Build history of the part. All positions in model axes, mm. A direction names the side the tool comes from. Round coordinates to 2 decimals unless told otherwise and drop trailing zeros. Write each loop counter-clockwise with the first axis right and the second up, starting at its lowest first coordinate (ties: lowest second). Pieces come first, ordered by that corner, then holes. Notation, with made-up numbers: (75.25, -32) - (101.25, -32) arc R15 cw to (101.25, -17) - close; hole circle Ø9 at (-35.75, 85.25). An arc over 180 degrees is marked (long way). One line per question, with ' | ' between items.
from build123d import *

# Parameters (mm, degrees)
SKETCH1_W               = 260
SKETCH1_H               = 150
SKETCH1_W_2             = 255
SKETCH1_H_2             = 145
BOSS_EXTRUDE1_DEPTH     = 110
SKETCH2_W               = 255
SKETCH2_H               = 145
BOSS_EXTRUDE2_DEPTH     = 2.5
SKETCH4_W               = 145
SKETCH4_H               = 2.5
BOSS_EXTRUDE3_DEPTH     = 45.5
CUT_EXTRUDE_THIN4_DEPTH = 5
SKETCH6_W               = 60
SKETCH6_H               = 30
CUT_EXTRUDE1_DEPTH      = 5
BOSS_EXTRUDE4_REACH     = 294.104
CUT_EXTRUDE2_DEPTH      = 3
SKETCH10_W              = 42.57
SKETCH10_H              = 23
CUT_EXTRUDE3_DEPTH      = 2.5
CUT_EXTRUDE4_DEPTH      = 2.5


with BuildPart() as part:
    # Sketch1 → Boss-Extrude1 (new body)
    with BuildSketch(Plane(origin=(0, 0, 0), x_dir=(1, 0, 0), z_dir=(0, 1, 0))):
        with Locations((130, 75)):
            Rectangle(SKETCH1_W, SKETCH1_H)
        with Locations((130, 75)):
            Rectangle(SKETCH1_W_2, SKETCH1_H_2, mode=Mode.SUBTRACT)
    extrude(amount=-BOSS_EXTRUDE1_DEPTH)

    # Sketch2 → Boss-Extrude2 (add)
    with BuildSketch(Plane(origin=(0, 0, 0), x_dir=(1, 0, 0), z_dir=(0, 1, 0))):
        with Locations((130, 75)):
            Rectangle(SKETCH2_W, SKETCH2_H)
    extrude(amount=-BOSS_EXTRUDE2_DEPTH)

    # Sketch4 → Boss-Extrude3 (add)
    with BuildSketch(Plane.ZY.offset(-257.5)):
        with Locations((-75, -93.15)):
            Rectangle(SKETCH4_W, SKETCH4_H)
    extrude(amount=BOSS_EXTRUDE3_DEPTH)

    # Sketch5 → Cut-Extrude-Thin4 (cut)
    with BuildSketch(Plane.XZ.offset(94.4)):
        Polygon((217.857864376, -60.857864376), (232, -75), (246.142135624, -60.857864376), (257.5, -60.857864376), (257.5, -60.858864376), (246.142549837, -60.858864376), (232, -75.001414214), (217.857157269, -60.858571483), align=None)
        with BuildLine():
            ThreePointArc((246.141113376, -60.858886624), (232, -55.001445677), (217.858886624, -60.858886624))
            Line((217.858886624, -60.858886624), (217.858179517, -60.858179517))
            ThreePointArc((217.858179517, -60.858179517), (232, -55.000445677), (246.141820483, -60.858179517))
            Line((246.141820483, -60.858179517), (246.141113376, -60.858886624))
        make_face()
    extrude(amount=-CUT_EXTRUDE_THIN4_DEPTH, mode=Mode.SUBTRACT)


with BuildPart() as cut_extrude_thin4_kept_piece:
    # of the separate pieces the step leaves, the one the design keeps (cut_extrude_thin4_pieces_kept)
    add(part.part.solids().sort_by_distance((0, 0, 0))[0])

    # Sketch6 → Cut-Extrude1 (cut)
    with BuildSketch(Plane(origin=(260, 0, 0), x_dir=(0, 0, -1), z_dir=(1, 0, 0))):
        with Locations((45, -78)):
            Rectangle(SKETCH6_W, SKETCH6_H)
    extrude(amount=-CUT_EXTRUDE1_DEPTH, mode=Mode.SUBTRACT)

    # Sketch8 → Boss-Extrude4 (add, up to next)
    with BuildSketch(Plane.XY.offset(-75), mode=Mode.PRIVATE) as boss_extrude4_sk1:
        Polygon((260, -63), (257.5, -64.647820306), (257.5, -63), align=None)
    boss_extrude4_tool1 = extrude(boss_extrude4_sk1.sketch, amount=BOSS_EXTRUDE4_REACH, mode=Mode.PRIVATE) - cut_extrude_thin4_kept_piece.part
    add(boss_extrude4_tool1.solids().sort_by_distance((258.333333, -63.549273, -75))[0])

    # Sketch9 → Cut-Extrude2 (cut)
    with BuildSketch(Plane.XZ.offset(94.4)):
        with BuildLine():
            Line((232, -75), (246.479283082, -87.467045982))
            ThreePointArc((246.479283082, -87.467045982), (232, -94.106984956), (217.520716918, -87.467045982))
            Line((217.520716918, -87.467045982), (232, -75))
        make_face()
    extrude(amount=-CUT_EXTRUDE2_DEPTH, mode=Mode.SUBTRACT)

    # Sketch10 → Cut-Extrude3 (cut)
    with BuildSketch(Plane(origin=(260, 0, 0), x_dir=(0, 0, -1), z_dir=(1, 0, 0))):
        with Locations((109.285, -44.84)):
            Rectangle(SKETCH10_W, SKETCH10_H)
    extrude(amount=-CUT_EXTRUDE3_DEPTH, mode=Mode.SUBTRACT)

    # Sketch11 → Cut-Extrude4 (cut)
    with BuildSketch(Plane(origin=(260, 0, 0), x_dir=(0, 0, -1), z_dir=(1, 0, 0))):
        Polygon((45, -93), (37.965, -93), (37.965, -110), (52.035, -110), (52.035, -93), align=None)
    extrude(amount=-CUT_EXTRUDE4_DEPTH, mode=Mode.SUBTRACT)


solid = cut_extrude_thin4_kept_piece.part
Q1. Saw through at D-D, the plane z = -72. List the corners of the cut face in (x, y), then the cut area to 3 significant figures.
Found:
outline: (0, -110) - (2.5, -110) - (2.5, -2.5) - (257.5, -2.5) - (257.5, -64.65) - (260, -63) - (260, 0) - (0, 0) - close; (212, -94.4) - (229, -94.4) - (229, -91.9) - (212, -91.9) - close; (235, -94.4) - (257.5, -94.4) - (257.5, -110) - (260, -110) - (260, -93) - (255, -93) - (255, -91.9) - (235, -91.9) - close | area: 1,210 mm^2
Q2. Saw through at B-B, the plane y = -6.5. List the corners of the cut face in (x, z).
Found:
outline: (0, -150) - (260, -150) - (260, 0) - (0, 0) - close; hole (2.5, -147.5) - (257.5, -147.5) - (257.5, -2.5) - (2.5, -2.5) - close
Q3. Saw through at A-A, the plane z = -34. List the corners of the cut face in (x, y), then the cut area to 3 significant figures.
Found:
outline: (0, -110) - (2.5, -110) - (2.5, -2.5) - (257.5, -2.5) - (257.5, -64.65) - (260, -63) - (260, 0) - (0, 0) - close; (212, -94.4) - (257.5, -94.4) - (257.5, -110) - (260, -110) - (260, -93) - (255, -93) - (255, -91.9) - (212, -91.9) - close | area: 1,230 mm^2
Q4. Which spindle directions (+Z, -Z, +X, -X, +Y, -Y) get a long thin tool onto all of the face, cutting with end or side? Do faces 5 (the flat face through (257.5, -101, -99)), 6 (the flat face through (128, -55, -147.5)), 7 (the flat face through (128, -54, -150)), 8 (the flat face through (259, -78, -15)), 9 (the flat face through (0, -54, -74)). Say none if no direction does.
Found:
face 5: -Y | face 6: none | face 7: -Z, +X, -X, +Y, -Y | face 8: +X | face 9: +Z, -Z, -X, +Y, -Y
Q5. Drill centre lines: L1, parallel to Z at x = 183, y = -38; L2, parallel to X at y = -34, z = -41; L3, parallel to Y at x = 212.5, z = -116. Where is each one in solid material? Low to high. Write a range as from..to.
Found:
L1: -150..-147.5, -2.5..0 | L2: 0..2.5, 257.5..260 | L3: -94.4..-91.9, -2.5..0
Q6. Saw through at C-C, the plane x = 171.5. List the corners of the cut face in (y, z).
Found:
outline: (-110, -150) - (0, -150) - (0, 0) - (-110, 0) - (-110, -2.5) - (-2.5, -2.5) - (-2.5, -147.5) - (-110, -147.5) - close
Q7. Drop flat-ended pins along their axis: pin 1 (6 mm diameter, centred on x = 123.5, z = -55.5, fed in from -Y); pin 2 (0.7 mm diameter, centred on y = -94, z = -44.5, fed in from +X). Give the stop position or say it passes through.
Found:
pin 1: y = -2.5 | pin 2: x = 257.5
Q8. Pull direction Y, two halves, no side cores. Call faces 1 (the flat face through (128, 0, -76)), 2 (the flat face through (260, -54, -74)), 3 (the flat face through (128, -55, -2.5)), 4 (the flat face through (257.5, -48, -76)): +Y half, -Y half, draft (parallel to the pull), parting line (faces both ways), or undercut.
Found:
face 1: +Y half | face 2: draft | face 3: undercut | face 4: undercut
